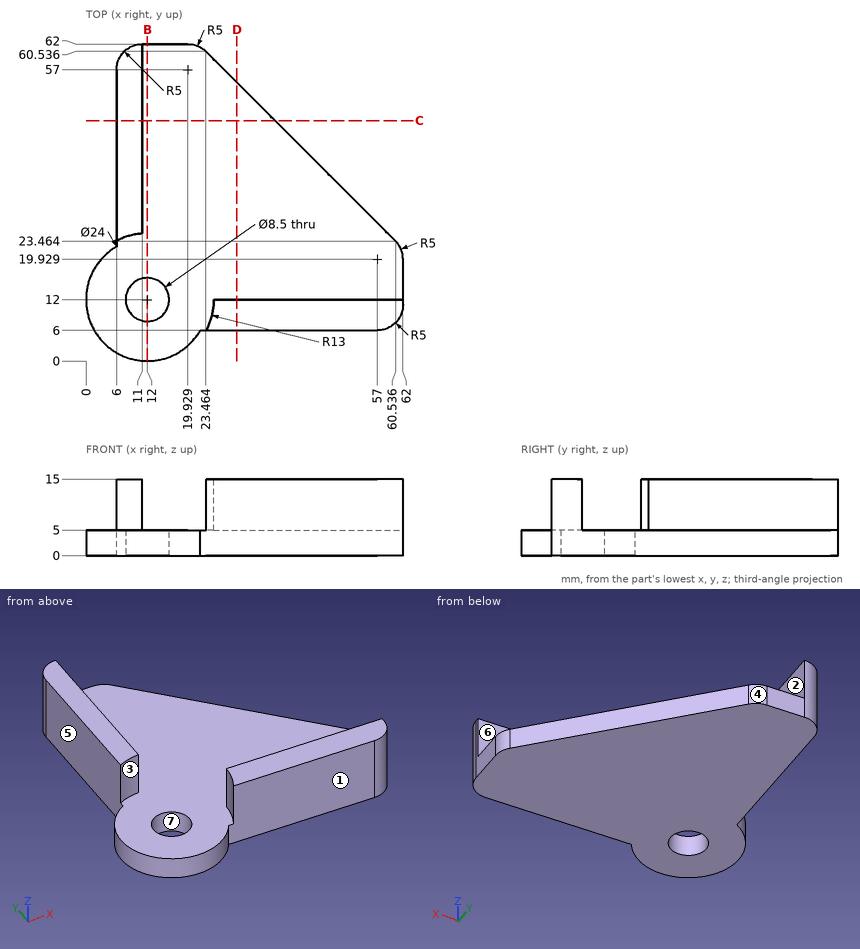
Here's the drawing with two shaded views (mm, measured from the low corner). I have some questions. A direction names the side the tool comes from. Round coordinates to 2 decimals unless told otherwise and drop trailing zeros. Write each loop counter-clockwise with the first axis right and the second up, starting at its lowest first coordinate (ties: lowest second). Pieces come first, ordered by that corner, then holes.
(1) For pin 1 (6 mm diameter, centred on x = 34, z = 12.5, fed in from +Y); pin 2 (7 mm diameter, centred on x = 12, y = 12, fed in from +Z); pin 3 (7.5 mm diameter, centred on y = 35.5, z = 9, fed in from -X); pin 4 (10 mm diameter, centred on x = 25, y = 42, fed in from +Z), each with a flat end and sliding along its axis, tell me the tip position at first contact or that it passes through.
Findings below:
pin 1: stops at y = 12
pin 2: passes through
pin 3: stops at x = 6
pin 4: stops at z = 5
(2) Which directions (+Z, -Z, +X, -X, +Y, -Y) give clear straight access to the entire face, cutting with the end or side of a thin tool? Please do the marked faces 1, 2 and 3.
Findings below:
face 1: +Z, -Z, +X, -Y
face 2: +Z, +X, +Y, -Y
face 3: +Z, +X, -Y
(3) Suppose I cut it at D-D on x = 29.5. Write out the boundary of the cut face in (y, z).
Findings below:
outline: (6, 0) - (54.5, 0) - (54.5, 5) - (12, 5) - (12, 15) - (6, 15) - close
(4) Suppose I cut it at B-B on x = 12. Write out the boundary of the cut face in (y, z).
Findings below:
outline: (0, 0) - (7.75, 0) - (7.75, 5) - (0, 5) - close; (16.25, 0) - (62, 0) - (62, 5) - (16.25, 5) - close
(5) Thinking about a two-plate mould opening in X: for the marked faces 4, 5, 6 and 7, which applies, +X half, -X half, draft (parallel to the pull), parting line (faces both ways), or undercut?
Findings below:
face 4: +X half
face 5: -X half
face 6: draft
face 7: undercut
(6) If I drill on probe 1 along Y at (x, z) = (12, 2.15); probe 2 along X at (y, z) = (30.5, 12.5); probe 3 along Y at (x, z) = (45, 6.25), over which ranges is the centre line in solid material (lowest first)?
Findings below:
probe 1: y = 0 to 7.75, 16.25 to 62
probe 2: x = 6 to 11
probe 3: y = 6 to 12
(7) Suppose I cut it at C-C on y = 47. Write out the boundary of the cut face in (x, z), and give its area (3 significant figures).
Findings below:
outline: (6, 0) - (37, 0) - (37, 5) - (11, 5) - (11, 15) - (6, 15) - close
area: 205 mm2
